```python
from build123d import *

# Parameters (mm, degrees)
BOSS_EXTRUDE2_DEPTH = 2
SKETCH3_W           = 735
SKETCH3_H           = 30
SKETCH3_W_2         = 30
SKETCH3_H_2         = 566.828478147
CUT_EXTRUDE1_DEPTH  = 0.5


with BuildPart() as part:
    # Sketch1 → Boss-Extrude2 (new body)
    with BuildSketch(Plane.XY):
        Polygon((381.097732077, 252.798507463), (-18.902267923, 252.798507463), (-18.902267923, 202.798507463), (-568.902267923, 202.798507463), (-568.902267923, -197.201492537), (-18.902267923, -197.201492537), (-18.902267923, -317.201492537), (381.097732077, -317.201492537), (381.097732077, -197.201492537), (431.097732077, -197.201492537), (431.097732077, 202.798507463), (381.097732077, 202.798507463), align=None)
    extrude(amount=BOSS_EXTRUDE2_DEPTH)

    # Sketch3 → Cut-Extrude1 (cut)
    with BuildSketch(Plane.XY.offset(2)):
        with Locations((-201.402267923, 2.798507463)):
            Rectangle(SKETCH3_W, SKETCH3_H)
        with Locations((181.097732077, -29.507440836)):
            Rectangle(SKETCH3_W_2, SKETCH3_H_2)
    extrude(amount=-CUT_EXTRUDE1_DEPTH, mode=Mode.SUBTRACT)


solid = part.part
```
Can you work these out from the model? Positions are in its coordinate system, mm. Give positions to 0.01 mm unless a question says otherwise; leave off trailing zeros. Order: outer loops, then holes, each group sorted by start corner. A loop starts at its lowest first (then second) coordinate and runs counter-clockwise, first axis right, second up. Notation, with made-up numbers: (-25, -27) - (32, -27) arc R9 cw to (32, -17) - close; hole circle Ø8 at (71, 57). An arc over 180 degrees is marked (long way). Use a Markdown table: item, result. Add a question column.
Q1. If we section it at C-C on x = -114: Write out the boundary of the cut face in (y, z).
Q2. If we section it at B-B on z = 1.1: Write out the boundary of the cut face in (x, y), plus the area to 3 significant figures.
Q3. I'm going to push flat-ended pins straight in: pin 1 (1 mm diameter, centred on x = -341.5, z = 0.5, fed in from +Y); pin 2 (1 mm diameter, centred on x = -163.5, z = 1, fed in from -Y); pin 3 (1 mm diameter, centred on y = 231.5, z = 1, fed in from -X); pin 4 (1 mm diameter, centred on x = 133.5, y = 134, fed in from -Z). Where does each tip first touch, or does it pass through?
Q4. Please list where these lines run through material, in increasing order: line 1 along X through (y, z) = (-249, 1.6); line 2 along Y through (x, z) = (-204, 1.85); line 3 along X through (y, z) = (8, 1.8).
Q5. If we section it at A-A on y = -256: Write out the boundary of the cut face in (x, z).
Answers follow:
| question | item | result |
|---|---|---|
| 1 | outline | (-197.2, 0) - (202.8, 0) - (202.8, 2) - (17.8, 2) - (17.8, 1.5) - (-12.2, 1.5) - (-12.2, 2) - (-197.2, 2) - close |
| 2 | outline | (-568.9, -197.2) - (-18.9, -197.2) - (-18.9, -317.2) - (381.1, -317.2) - (381.1, -197.2) - (431.1, -197.2) - (431.1, 202.8) - (381.1, 202.8) - (381.1, 252.8) - (-18.9, 252.8) - (-18.9, 202.8) - (-568.9, 202.8) - close |
| 2 | area | 468,000 mm^2 |
| 3 | pin 1 | stops at y = 202.8 |
| 3 | pin 2 | stops at y = -197.2 |
| 3 | pin 3 | stops at x = -18.9 |
| 3 | pin 4 | stops at z = 0 |
| 4 | line 1 | x = -18.9 to 166.1, 196.1 to 381.1 |
| 4 | line 2 | y = -197.2 to -12.2, 17.8 to 202.8 |
| 4 | line 3 | x = 196.1 to 431.1 |
| 5 | outline | (-18.9, 0) - (381.1, 0) - (381.1, 2) - (196.1, 2) - (196.1, 1.5) - (166.1, 1.5) - (166.1, 2) - (-18.9, 2) - close |
